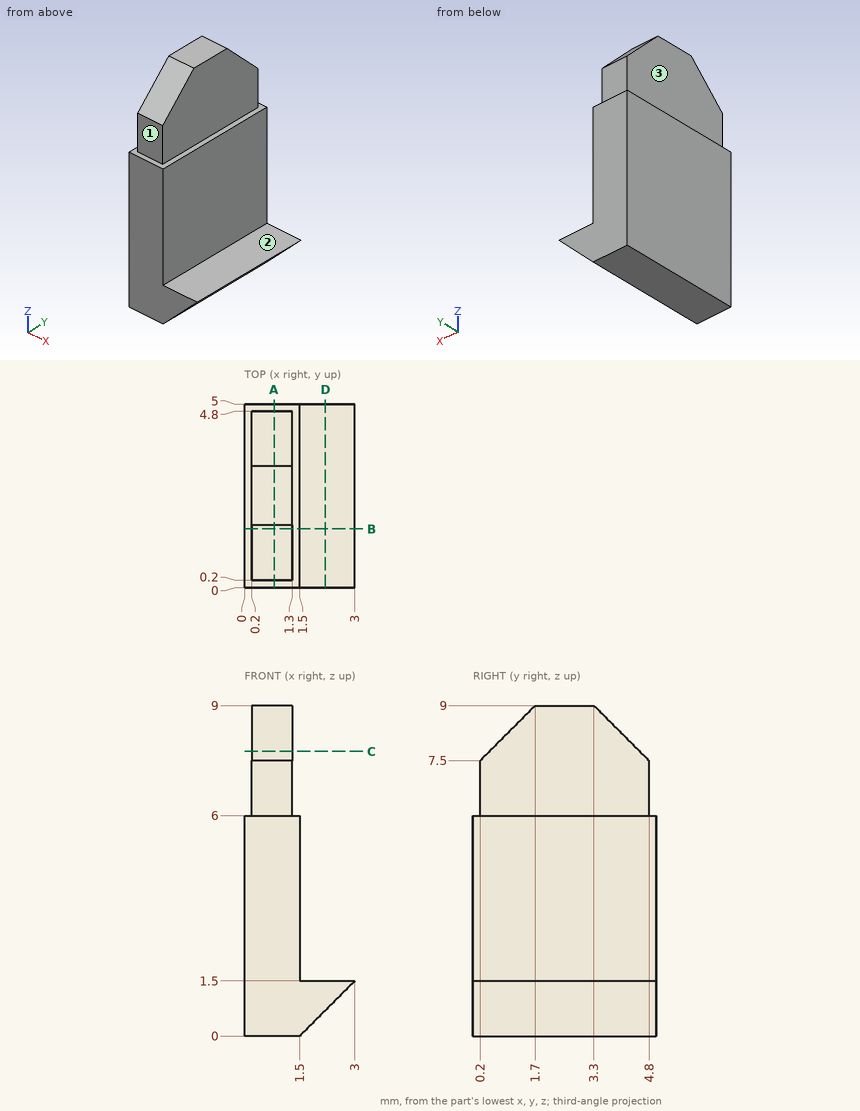
Verification items for this drawing (mm, ordinates from the low corner). A direction names the side the tool comes from. Coordinates: 2 decimals unless noted, no trailing zeros. Loops run counter-clockwise (first coordinate to the right, second up) from the corner with the lowest first, then second, coordinate; pieces in that order, holes last. Notation, with made-up numbers: (-28.75, 26) - (-0.75, 26) arc R31 ccw to (-0.75, 54) - close; hole circle Ø10 at (28.25, 26). An arc over 180 degrees is marked (long way). Answer as a JSON object with one key per item and string values.
(1) Cross-section at D-D, the plane x = 2.2. Record the boundary of the cut face in (y, z).
Response:
{"outline": "(0, 0.7) - (5, 0.7) - (5, 1.5) - (0, 1.5) - close"}
(2) Go/stop test with flat-tipped pins: pin 1 Ø0.9 at (y, z) = (1.5, 8) entering from +X; pin 2 Ø0.9 at (x, z) = (0.5, 7) entering from +Y; pin 3 Ø1 at (y, z) = (2.5, 5.5) entering from +X. Record where each tip stops, or that it passes through.
Response:
{"pin 1": "stops at x = 1.3", "pin 2": "stops at y = 4.8", "pin 3": "stops at x = 1.5"}
(3) Cross-section at B-B, the plane y = 1.6. Record the boundary of the cut face in (x, z), then the cut area to 3 significant figures.
Response:
{"outline": "(0, 0) - (1.5, 0) - (3, 1.5) - (1.5, 1.5) - (1.5, 6) - (1.3, 6) - (1.3, 8.9) - (0.2, 8.9) - (0.2, 6) - (0, 6) - close", "area": "13.3 mm²"}
(4) Access from +Z, -Z, +X, -X, +Y, -Y to the whole of each face (thin tool, end or side, straight path). Record for the marked faces 1, 2 and 3.
Response:
{"face 1": "+Z, +X, -X, -Y", "face 2": "+Z, +X, +Y, -Y", "face 3": "+Z, -X, +Y, -Y"}
(5) Cross-section at A-A, the plane x = 0.8. Record the boundary of the cut face in (y, z).
Response:
{"outline": "(0, 0) - (5, 0) - (5, 6) - (4.8, 6) - (4.8, 7.5) - (3.3, 9) - (1.7, 9) - (0.2, 7.5) - (0.2, 6) - (0, 6) - close"}
(6) Scan lines: line 1 along X through (y, z) = (2.8, 6.5); line 2 along Z through (x, y) = (1.45, 0.9); line 3 along X through (y, z) = (4.55, 3.5). Record each from-to range of solid material in increasing order.
Response:
{"line 1": "x = 0.2 to 1.3", "line 2": "z = 0 to 6", "line 3": "x = 0 to 1.5"}
(7) Cross-section at C-C, the plane z = 7.75. Record the boundary of the cut face in (x, y), then the cut area to 3 significant figures.
Response:
{"outline": "(0.2, 0.45) - (1.3, 0.45) - (1.3, 4.55) - (0.2, 4.55) - close", "area": "4.51 mm²"}
